from build123d import *

# Parameters (mm, degrees)
F0_R     = 6.35
F1_DEPTH = 3.175


with BuildPart() as f1:
    # F0 (on Right) → F1 (new body)
    with BuildSketch(Plane.YZ):
        with BuildLine():
            Line((0, 152.4), (0, 0))
            Line((0, 0), (0, -82.55))
            Line((0, -82.55), (6.35, -82.55))
            ThreePointArc((6.35, -82.55), (12.7, -76.2), (19.05, -82.55))
            Line((19.05, -82.55), (25.4, -82.55))
            Line((25.4, -82.55), (25.4, -9.525))
            Line((25.4, -9.525), (25.4, 6.007355))
            Line((25.4, 6.007355), (25.4, 152.4))
            ThreePointArc((25.4, 152.4), (12.7, 165.1), (0, 152.4))
        make_face()
        with Locations((12.7, -6.35)):
            Circle(F0_R, mode=Mode.SUBTRACT)
        with Locations((12.7, 152.4)):
            Circle(F0_R, mode=Mode.SUBTRACT)
        with BuildLine():
            Line((6.35, -82.55), (0, -82.55))
            ThreePointArc((0, -82.55), (12.7, -95.25), (25.4, -82.55))
            Line((25.4, -82.55), (19.05, -82.55))
            ThreePointArc((19.05, -82.55), (12.7, -88.9), (6.35, -82.55))
        make_face()
    extrude(amount=F1_DEPTH)


solid = f1.part
The model under review builds one solid part; all positions refer to its coordinate system, in mm. Coordinates: 2 decimals unless noted, no trailing zeros. Write each loop counter-clockwise with the first axis right and the second up, starting at its lowest first coordinate (ties: lowest second). Pieces come first, ordered by that corner, then holes. Notation, with made-up numbers: (-8, 22) -> (24, 22) arc R28 ccw to (24, 51) -> close; hole circle Ø5 at (68.25, 29.25). An arc over 180 degrees is marked (long way). Answer in a Markdown table with one row per item.
1. We need section D-D, the plane y = 3.5. State the section outline as (x, z) points (3 decimals), and give its area (3 significant figures).
Answers below:
| item | result |
|---|---|
| outline | (0, -91.305) -> (3.175, -91.305) -> (3.175, 161.155) -> (0, 161.155) -> close |
| area | 802 mm^2 |
2. We need section C-C, the plane y = 12.7. State the section outline as (x, z) points (3 decimals).
Answers below:
| item | result |
|---|---|
| outline | (0, -95.25) -> (3.175, -95.25) -> (3.175, -88.9) -> (0, -88.9) -> close; (0, -76.2) -> (3.175, -76.2) -> (3.175, -12.7) -> (0, -12.7) -> close; (0, 0) -> (3.175, 0) -> (3.175, 146.05) -> (0, 146.05) -> close; (0, 158.75) -> (3.175, 158.75) -> (3.175, 165.1) -> (0, 165.1) -> close |
3. We need section B-B, the plane x = 0.75. State the section outline as (y, z) points, and give its area (3 significant figures).
Answers below:
| item | result |
|---|---|
| outline | (0, -82.55) arc R12.7 ccw to (25.4, -82.55) -> (25.4, 152.4) arc R12.7 ccw to (0, 152.4) -> close; hole circle Ø12.7 at (12.7, -82.55); hole circle Ø12.7 at (12.7, -6.35); hole circle Ø12.7 at (12.7, 152.4) |
| area | 6,090 mm^2 |
4. Clearance check with a flat-ended pin moving along its axis: pin 1 Ø6 at (y, z) = (9, 93.5) entering from -X. State where the tip first meets the part, or that it passes through.
Answers below:
| item | result |
|---|---|
| pin 1 | stops at x = 0 |
5. We need section A-A, the plane z = -6.35. State the section outline as (x, y) points (3 decimals), and give its area (3 significant figures).
Answers below:
| item | result |
|---|---|
| outline | (0, 0) -> (3.175, 0) -> (3.175, 6.35) -> (0, 6.35) -> close; (0, 19.05) -> (3.175, 19.05) -> (3.175, 25.4) -> (0, 25.4) -> close |
| area | 40.3 mm^2 |
6. Draft analysis for pull direction Z (two halves, no side actions). For faces 1 (the flat face through (3.175, 13, 37)), 2 (the cylindrical face through (1.57, 8.02, -86.84)), 3 (the cylindrical face through (1.57, 7.66, -10.21)), 4 (the cylindrical face through (1.565, 12.979, 165.097)), state which applies: +Z half, -Z half, draft (parallel to the pull), parting line (faces both ways), or undercut.
Answers below:
| item | result |
|---|---|
| face 1 | draft |
| face 2 | undercut |
| face 3 | undercut |
| face 4 | +Z half |
7. Wall thickness on probe 1 along Z at (x, y) = (2.3, 12.7); probe 2 along Y at (x, z) = (1.85, -82.55); probe 3 along Z at (x, y) = (1.8, 16.5): over which ranges is each line inside the solid? List them lowest first. Write a range as [from, to].
Answers below:
| item | result |
|---|---|
| probe 1 | z = [-95.25, -88.9], [-76.2, -12.7], [0, 146.05], [158.75, 165.1] |
| probe 2 | y = [0, 6.35], [19.05, 25.4] |
| probe 3 | z = [-94.67, -87.64], [-77.46, -11.44], [-1.26, 147.31], [157.49, 164.52] |
